The model under review builds one solid part; all positions refer to its coordinate system, in mm. Face numbers are marked on the shaded views. Round coordinates to 2 decimals unless told otherwise and drop trailing zeros. Write each loop counter-clockwise with the first axis right and the second up, starting at its lowest first coordinate (ties: lowest second). Pieces come first, ordered by that corner, then holes. Notation, with made-up numbers: M 57.25,22 L 70.25,22 A23 cw 70.25,49 Z; hole C 19,-29.75 d3. An arc over 180 degrees is marked long. One line per item, written item: value. Start each with the question number.
1) For P1, Ø1.6, axis at x = 0, y = 5, coming from the -Z side; P2, Ø2.5, axis at x = -1, z = -0.5, coming from the +Y side; P3, Ø3, axis at y = 5.5, z = -16.5, coming from the -X side; P4, Ø4, axis at y = 6.5, z = -14, coming from the +X side, all flat-tipped, find the tip position at first contact; note any pin that passes through.
2) Take a section at C-C, the plane y = 0.75. Write out the cut boundary in (x, z), and give its area (3 significant figures).
3) Take a section at A-A, the plane y = 5. Write out the cut boundary in (x, z).
4) Take a section at D-D, the plane z = 11. Write out the cut boundary in (x, y), and give its area (3 significant figures).
5) Mouldability with a two-part tool opening along Z and no side actions: class the marked faces 1, 2 and 3 as +Z half, -Z half, draft (parallel to the pull), parting line (faces both ways), or undercut.
6) Take a section at B-B, the plane z = 0. Write out the cut boundary in (x, y).
7) Wall thickness on probe 1 along X at (y, z) = (6.5, 0); probe 2 along Z at (x, y) = (7.5, 1.75); probe 3 along X at (y, z) = (5.25, 3): over which ranges is each line inside the solid? List them lowest first.
from build123d import *

# Parameters (mm, degrees)
SKETCH2_R               = 20
BOSS_EXTRUDE1_DEPTH     = 8
CUT_EXTRUDE7_DEPTH      = 33.622844756
CUT_EXTRUDE7_DEPTH_BACK = 33.622844756
SKETCH7_R               = 1
CUT_EXTRUDE8_DEPTH      = 13.5
CUT_EXTRUDE15_DEPTH     = 15
SKETCH3_R               = 4.5
CUT_EXTRUDE16_DEPTH     = 6
SKETCH12_R              = 1.5
CUT_EXTRUDE17_DEPTH     = 3


with BuildPart() as part:
    # Sketch2 → Boss-Extrude1 (new body)
    with BuildSketch(Plane(origin=(0, 0, 0), x_dir=(1, 0, 0), z_dir=(0, 1, 0))):
        with Locations(Location((0, 0, 0), (0, 0, 270))):
            Circle(SKETCH2_R)
    extrude(amount=BOSS_EXTRUDE1_DEPTH)

    # Sketch7 → Cut-Extrude7 (cut, two sides: drawn at the far end of the back side and taken through both)
    with BuildSketch(Plane.XY.offset(4.5).offset(-CUT_EXTRUDE7_DEPTH_BACK)):
        with Locations(Location((0, 5, 0), (0, 0, 90))):
            Circle(SKETCH7_R)
    extrude(amount=CUT_EXTRUDE7_DEPTH + CUT_EXTRUDE7_DEPTH_BACK, mode=Mode.SUBTRACT)

    # Sketch9 → Cut-Extrude8 (cut)
    with BuildSketch(Plane.XY.offset(20)):
        with BuildLine():
            Line((2.5, 4.5), (2.5, 8))
            Line((2.5, 8), (-2.5, 8))
            Line((-2.5, 8), (-2.5, 4.5))
            ThreePointArc((-2.5, 4.5), (0, 2), (2.5, 4.5))
        make_face()
    extrude(amount=-CUT_EXTRUDE8_DEPTH, mode=Mode.SUBTRACT)

    # Sketch10 → Cut-Extrude15 (cut)
    with BuildSketch(Plane.XY.offset(-6.5)):
        with BuildLine():
            Line((0, 8), (0, 2))
            ThreePointArc((0, 2), (1.767766953, 2.732233047), (2.5, 4.5))
            Line((2.5, 4.5), (2.5, 8))
            Line((2.5, 8), (0, 8))
        make_face()
        with BuildLine():
            ThreePointArc((-2.5, 4.5), (-1.767766953, 2.732233047), (0, 2))
            Line((0, 2), (0, 8))
            Line((0, 8), (-2.5, 8))
            Line((-2.5, 8), (-2.5, 4.5))
        make_face()
    extrude(amount=-CUT_EXTRUDE15_DEPTH, mode=Mode.SUBTRACT)

    # Sketch3 → Cut-Extrude16 (cut)
    with BuildSketch(Plane(origin=(0, 8, 0), x_dir=(1, 0, 0), z_dir=(0, 1, 0))):
        with Locations(Location((0, 0, 0), (0, 0, 270))):
            Circle(SKETCH3_R)
    extrude(amount=-CUT_EXTRUDE16_DEPTH, mode=Mode.SUBTRACT)

    # Sketch12 → Cut-Extrude17 (cut)
    with BuildSketch(Plane.XZ):
        with Locations(Location((-8.485281374, 8.485281374, 0), (0, 0, 270))):
            Circle(SKETCH12_R)
        with Locations(Location((8.485281374, 8.485281374, 0), (0, 0, 270))):
            Circle(SKETCH12_R)
        with Locations(Location((8.485281374, -8.485281374, 0), (0, 0, 270))):
            Circle(SKETCH12_R)
        with Locations(Location((-8.485281374, -8.485281374, 0), (0, 0, 270))):
            Circle(SKETCH12_R)
    extrude(amount=-CUT_EXTRUDE17_DEPTH, mode=Mode.SUBTRACT)


solid = part.part
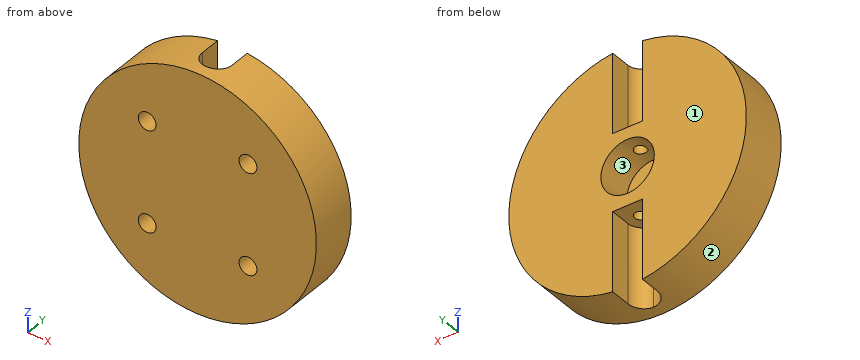
Checked values:
1. P1: passes through
1. P2: stops at y = 2
1. P3: stops at x = -13.23
1. P4: stops at x = 16
2. outline: C 0,0 d40; hole C -8.49,-8.49 d3; hole C -8.49,8.49 d3; hole C 8.49,-8.49 d3; hole C 8.49,8.49 d3
2. area: 1,230 mm2
3. outline: M -2.5,-19.84 L -2.5,-6.5 L -1,-6.5 L -1,-4.39 A4.5 cw -1,4.39 L -1,6.5 L -2.5,6.5 L -2.5,19.84 A20 ccw Z; M 1,-6.5 L 2.5,-6.5 L 2.5,-19.84 A20 ccw 2.5,19.84 L 2.5,6.5 L 1,6.5 L 1,4.39 A4.5 cw 1,-4.39 Z
4. outline: M -16.7,0 L 16.7,0 L 16.7,8 L 2.5,8 L 2.5,4.5 A2.5 cw -2.5,4.5 L -2.5,8 L -16.7,8 Z
4. area: 240 mm2
5. face 1: draft
5. face 2: parting line
5. face 3: undercut
6. outline: M -20,0 L 20,0 L 20,8 L 4.5,8 L 4.5,2 L -4.5,2 L -4.5,8 L -20,8 Z
7. probe 1: x = -20 to -4.5, 4.5 to 20
7. probe 2: z = -18.54 to -9.62, -7.35 to 7.35, 9.62 to 18.54
7. probe 3: x = -19.77 to -3.35, 3.35 to 19.77
